Check sheet for the modelled part. Datum: model origin and axes. Units: mm. A direction names the side the tool comes from. Give positions to 0.01 mm unless a question says otherwise; leave off trailing zeros. Loops run counter-clockwise (first coordinate to the right, second up) from the corner with the lowest first, then second, coordinate; pieces in that order, holes last. Notation, with made-up numbers: (25.5, -27) - (64.5, -27) arc R29 cw to (64.5, 7) - close; hole circle Ø7 at (-21.5, 70.5). An arc over 180 degrees is marked (long way). Use CSV: the item, a comma, the result in double quotes.
from build123d import *

# Parameters (mm, degrees)
F1_DEPTH = 2.54
F2_DEPTH = 10.16
F3_DEPTH = 2.54
F4_DEPTH = 15.24


with BuildPart() as f1:
    # F0 (on Top) → F1 (new body)
    with BuildSketch(Plane.XY):
        with BuildLine():
            Line((4.6571345698, 30.12210978), (12.7, 82.1429547439))
            ThreePointArc((12.7, 82.1429547439), (6.5740037456, 79.6054840123), (0, 78.74))
            Line((0, 78.74), (0, 30.48))
            ThreePointArc((0, 30.48), (2.3354329262, 30.3903957369), (4.6571345698, 30.12210978))
        make_face()
        with BuildLine():
            Line((12.7, 57.15), (12.7, 82.1429547439))
            Line((12.7, 82.1429547439), (4.6571345698, 30.12210978))
            ThreePointArc((4.6571345698, 30.12210978), (8.7620977053, 29.1934246673), (12.7, 27.7081287712))
            Line((12.7, 27.7081287712), (12.7, 57.15))
        make_face()
        with BuildLine():
            Line((1.9635281017, 12.7), (4.6571345698, 30.12210978))
            ThreePointArc((4.6571345698, 30.12210978), (2.3354329262, 30.3903957369), (0, 30.48))
            Line((0, 30.48), (0, 12.7))
            Line((0, 12.7), (1.9635281017, 12.7))
        make_face()
        with BuildLine():
            Line((0.9702363687, 6.2754395375), (1.9635281017, 12.7))
            Line((1.9635281017, 12.7), (0, 12.7))
            Line((0, 12.7), (0, 6.35))
            ThreePointArc((0, 6.35), (0.4865485263, 6.3313324452), (0.9702363687, 6.2754395375))
        make_face()
        with BuildLine():
            Line((0.3880945475, 2.510175815), (0.9702363687, 6.2754395375))
            ThreePointArc((0.9702363687, 6.2754395375), (0.4865485263, 6.3313324452), (0, 6.35))
            Line((0, 6.35), (0, 2.54))
            ThreePointArc((0, 2.54), (0.1946194105, 2.5325329781), (0.3880945475, 2.510175815))
        make_face()
        with BuildLine():
            Line((2.510175815, 0.3880945475), (6.2754395375, 0.9702363687))
            ThreePointArc((6.2754395375, 0.9702363687), (4.4901280605, 4.4901280605), (0.9702363687, 6.2754395375))
            Line((0.9702363687, 6.2754395375), (0.3880945475, 2.510175815))
            ThreePointArc((0.3880945475, 2.510175815), (1.7960512242, 1.7960512242), (2.510175815, 0.3880945475))
        make_face()
        with BuildLine():
            Line((2.54, 0), (6.35, 0))
            ThreePointArc((6.35, 0), (6.3313324452, 0.4865485263), (6.2754395375, 0.9702363687))
            Line((6.2754395375, 0.9702363687), (2.510175815, 0.3880945475))
            ThreePointArc((2.510175815, 0.3880945475), (2.5325329781, 0.1946194105), (2.54, 0))
        make_face()
        with BuildLine():
            Line((6.35, 0), (12.7, 0))
            Line((12.7, 0), (12.7, 1.9635281017))
            Line((12.7, 1.9635281017), (6.2754395375, 0.9702363687))
            ThreePointArc((6.2754395375, 0.9702363687), (6.3313324452, 0.4865485263), (6.35, 0))
        make_face()
        with BuildLine():
            Line((12.7, 0), (30.48, 0))
            ThreePointArc((30.48, 0), (30.3903957369, 2.3354329262), (30.12210978, 4.6571345698))
            Line((30.12210978, 4.6571345698), (12.7, 1.9635281017))
            Line((12.7, 1.9635281017), (12.7, 0))
        make_face()
        with BuildLine():
            Line((30.48, 0), (78.74, 0))
            ThreePointArc((78.74, 0), (79.6054840123, 6.5740037456), (82.1429547439, 12.7))
            Line((82.1429547439, 12.7), (30.12210978, 4.6571345698))
            ThreePointArc((30.12210978, 4.6571345698), (30.3903957369, 2.3354329262), (30.48, 0))
        make_face()
        with BuildLine():
            Line((27.7081287712, 12.7), (57.15, 12.7))
            ThreePointArc((57.15, 12.7), (25.7191035763, 25.7191035763), (12.7, 57.15))
            Line((12.7, 57.15), (12.7, 27.7081287712))
            ThreePointArc((12.7, 27.7081287712), (21.5526146906, 21.5526146906), (27.7081287712, 12.7))
        make_face()
        with BuildLine():
            Line((30.12210978, 4.6571345698), (82.1429547439, 12.7))
            Line((82.1429547439, 12.7), (57.15, 12.7))
            Line((57.15, 12.7), (27.7081287712, 12.7))
            ThreePointArc((27.7081287712, 12.7), (29.1934246673, 8.7620977053), (30.12210978, 4.6571345698))
        make_face()
        with BuildLine():
            Line((126.1370452561, 12.7), (134.0196045361, 12.7))
            ThreePointArc((134.0196045361, 12.7), (95.1907148833, 95.1907148833), (12.7, 134.0196045361))
            Line((12.7, 134.0196045361), (12.7, 126.1370452561))
            ThreePointArc((12.7, 126.1370452561), (21.9970452561, 116.84), (25.4, 104.14))
            ThreePointArc((25.4, 104.14), (21.9970452561, 91.44), (12.7, 82.1429547439))
            Line((12.7, 82.1429547439), (12.7, 57.15))
            ThreePointArc((12.7, 57.15), (57.15, 101.6), (101.6, 57.15))
            ThreePointArc((101.6, 57.15), (88.5808964237, 25.7191035763), (57.15, 12.7))
            Line((57.15, 12.7), (82.1429547439, 12.7))
            ThreePointArc((82.1429547439, 12.7), (104.14, 25.4), (126.1370452561, 12.7))
        make_face()
        with BuildLine():
            Line((129.54, 0), (134.62, 0))
            ThreePointArc((134.62, 0), (134.4698173618, 6.3570919986), (134.0196045361, 12.7))
            Line((134.0196045361, 12.7), (126.1370452561, 12.7))
            ThreePointArc((126.1370452561, 12.7), (128.6745159877, 6.5740037456), (129.54, 0))
        make_face()
        with BuildLine():
            Line((12.7, 126.1370452561), (12.7, 134.0196045361))
            ThreePointArc((12.7, 134.0196045361), (6.3570919986, 134.4698173618), (0, 134.62))
            Line((0, 134.62), (0, 129.54))
            ThreePointArc((0, 129.54), (6.5740037456, 128.6745159877), (12.7, 126.1370452561))
        make_face()
        with BuildLine():
            Line((82.1429547439, 12.7), (126.1370452561, 12.7))
            ThreePointArc((126.1370452561, 12.7), (104.14, 25.4), (82.1429547439, 12.7))
        make_face()
        with BuildLine():
            Line((78.74, 0), (129.54, 0))
            ThreePointArc((129.54, 0), (128.6745159877, 6.5740037456), (126.1370452561, 12.7))
            Line((126.1370452561, 12.7), (82.1429547439, 12.7))
            ThreePointArc((82.1429547439, 12.7), (79.6054840123, 6.5740037456), (78.74, 0))
        make_face()
    extrude(amount=F1_DEPTH)

    # F0 (on Top) → F2 (join)
    with BuildSketch(Plane.XY):
        with BuildLine():
            ThreePointArc((134.0196045361, 12.7), (134.4698173618, 6.3570919986), (134.62, 0))
            Line((134.62, 0), (137.16, 0))
            ThreePointArc((137.16, 0), (137.0126136617, 6.3568307817), (136.5707713971, 12.7))
            Line((136.5707713971, 12.7), (134.0196045361, 12.7))
        make_face()
        with BuildLine():
            ThreePointArc((12.7, 134.0196045361), (95.1907148833, 95.1907148833), (134.0196045361, 12.7))
            Line((134.0196045361, 12.7), (136.5707713971, 12.7))
            ThreePointArc((136.5707713971, 12.7), (96.9867661075, 96.9867661075), (12.7, 136.5707713971))
            Line((12.7, 136.5707713971), (12.7, 134.0196045361))
        make_face()
        with BuildLine():
            ThreePointArc((0, 134.62), (6.3570919986, 134.4698173618), (12.7, 134.0196045361))
            Line((12.7, 134.0196045361), (12.7, 136.5707713971))
            ThreePointArc((12.7, 136.5707713971), (6.3568307817, 137.0126136617), (0, 137.16))
            Line((0, 137.16), (0, 134.62))
        make_face()
    extrude(amount=F2_DEPTH)

    # F0 (on Top) → F3 (join)
    with BuildSketch(Plane.XY):
        with BuildLine():
            ThreePointArc((136.5707713971, 12.7), (137.0126136617, 6.3568307817), (137.16, 0))
            Line((137.16, 0), (142.24, 0))
            ThreePointArc((142.24, 0), (142.0979043334, 6.3563499), (141.6719012366, 12.7))
            Line((141.6719012366, 12.7), (136.5707713971, 12.7))
        make_face()
        with BuildLine():
            ThreePointArc((12.7, 136.5707713971), (96.9867661075, 96.9867661075), (136.5707713971, 12.7))
            Line((136.5707713971, 12.7), (141.6719012366, 12.7))
            ThreePointArc((141.6719012366, 12.7), (100.578868556, 100.578868556), (12.7, 141.6719012366))
            Line((12.7, 141.6719012366), (12.7, 136.5707713971))
        make_face()
        with BuildLine():
            ThreePointArc((0, 137.16), (6.3568307817, 137.0126136617), (12.7, 136.5707713971))
            Line((12.7, 136.5707713971), (12.7, 141.6719012366))
            ThreePointArc((12.7, 141.6719012366), (6.3563499, 142.0979043334), (0, 142.24))
            Line((0, 142.24), (0, 137.16))
        make_face()
    extrude(amount=F3_DEPTH)

    # F0 (on Top) → F4 (join)
    with BuildSketch(Plane.XY):
        with BuildLine():
            ThreePointArc((12.7, 141.6719012366), (100.578868556, 100.578868556), (141.6719012366, 12.7))
            Line((141.6719012366, 12.7), (144.2219067964, 12.7))
            ThreePointArc((144.2219067964, 12.7), (102.3749197802, 102.3749197802), (12.7, 144.2219067964))
            Line((12.7, 144.2219067964), (12.7, 141.6719012366))
        make_face()
        with BuildLine():
            ThreePointArc((0, 142.24), (6.3563499, 142.0979043334), (12.7, 141.6719012366))
            Line((12.7, 141.6719012366), (12.7, 144.2219067964))
            ThreePointArc((12.7, 144.2219067964), (6.3561283031, 144.6404094055), (0, 144.78))
            Line((0, 144.78), (0, 142.24))
        make_face()
        with BuildLine():
            ThreePointArc((141.6719012366, 12.7), (142.0979043334, 6.3563499), (142.24, 0))
            Line((142.24, 0), (144.78, 0))
            ThreePointArc((144.78, 0), (144.6404094055, 6.3561283031), (144.2219067964, 12.7))
            Line((144.2219067964, 12.7), (141.6719012366, 12.7))
        make_face()
    extrude(amount=F4_DEPTH)


solid = f1.part
1. Sectioned sample at C-C, the plane x = 120.5. Record the boundary of the cut face in (y, z).
Completed:
outline,"(0, 0) - (80.26, 0) - (80.26, 15.24) - (75.58, 15.24) - (75.58, 2.54) - (65.52, 2.54) - (65.52, 10.16) - (60.02, 10.16) - (60.02, 2.54) - (0, 2.54) - close"
2. Go/stop test with flat-tipped pins: pin 1 Ø5 at (y, z) = (119.5, 8.5) entering from +X; pin 2 Ø1 at (y, z) = (55.5, 11.5) entering from -X; pin 3 Ø1 at (y, z) = (129.5, 13.5) entering from -X. Record where each tip stops, or that it passes through.
Completed:
pin 1,"stops at x = 85.28"
pin 2,"stops at x = 130.75"
pin 3,"stops at x = 57.73"
3. Scan lines: line 1 along Z through (x, y) = (32, 13); line 2 along X through (y, z) = (33.5, 6); line 3 along X through (y, z) = (67.5, 7.5). Record each from-to range of solid material in increasing order.
Completed:
line 1,"z = 0 to 2.54"
line 2,"x = 130.39 to 133.01, 138.24 to 140.85"
line 3,"x = 116.47 to 119.4, 125.2 to 128.08"
4. Release check for a two-part mould opening along X. For faces 4 (the face through (79, 0, 2)), 5 (the face through (97, 98, 2.54)), 6 (the face through (0, 139, 2)) record: released by +X, released by -X, zero draft, split by the parting line, or undercut.
Completed:
face 4,"zero draft"
face 5,"undercut"
face 6,"released by -X"
5. Sectioned sample at A-A, the plane z = 6.5. Record the boundary of the cut face in (x, y), and give its area (3 significant figures).
Completed:
outline,"(0, 134.62) arc R134.62 cw to (134.62, 0) - (137.16, 0) arc R137.16 ccw to (0, 137.16) - close; (0, 142.24) arc R142.24 cw to (142.24, 0) - (144.78, 0) arc R144.78 ccw to (0, 144.78) - close"
area,"1,110 mm²"
6. Set-up check for faces 1 (the face through (93.5, 110.3, 15.24)), 2 (the face through (4.53, 4.45, 1.25)), 3 (the face through (89, 104, 10.16)): record each of +Z, -Z, +X, -X, +Y, -Y from which the full face is reachable in a straight line by a thin tool's end or side.
Completed:
face 1,"+Z, +X, -X, +Y, -Y"
face 2,"+Z, -Z"
face 3,"+Z, -X, -Y"
7. Sectioned sample at D-D, the plane y = 24.5. Record the boundary of the cut face in (x, z), and give its area (3 significant figures).
Completed:
outline,"(0, 0) - (3.79, 0) - (3.79, 2.54) - (0, 2.54) - close; (18.13, 0) - (26.99, 0) - (26.99, 2.54) - (18.13, 2.54) - close; (87.31, 0) - (142.69, 0) - (142.69, 15.24) - (140.11, 15.24) - (140.11, 2.54) - (134.95, 2.54) - (134.95, 10.16) - (132.37, 10.16) - (132.37, 2.54) - (87.31, 2.54) - close"
area,"225 mm²"
8. Sectioned sample at B-B, the plane y = 64. Record the boundary of the cut face in (x, z), and give its area (3 significant figures).
Completed:
outline,"(0, 0) - (13.23, 0) - (13.23, 2.54) - (0, 2.54) - close; (101.07, 0) - (129.87, 0) - (129.87, 15.24) - (127.03, 15.24) - (127.03, 2.54) - (121.31, 2.54) - (121.31, 10.16) - (118.43, 10.16) - (118.43, 2.54) - (101.07, 2.54) - close"
area,"165 mm²"
